```python
from build123d import *

# Parameters (mm, degrees)
SKETCH_R             = 2.5
PAD_DEPTH            = 4.7
SKETCH_MIRRORED_2_R  = 2.5
PAD_MIRRORED_2_DEPTH = 4.7


with BuildPart() as part:
    # Sketch → Pad (new body)
    with BuildSketch(Plane.XY):
        with BuildLine():
            Line((0, 0), (28.25, 0))
            Line((28.25, 0), (28.25, 23.538582))
            ThreePointArc((28.25, 23.538582), (26.870058, 26.870058), (23.538582, 28.25))
            Line((23.538582, 28.25), (0, 28.25))
            Line((0, 28.25), (0, 0))
        make_face()
        with Locations((23.5, 23.5)):
            Circle(SKETCH_R, mode=Mode.SUBTRACT)
    pad = extrude(amount=PAD_DEPTH)

    # Sketch Mirrored 2 → Pad Mirrored 2 (add)
    with BuildSketch(Plane(origin=(0, 0, 0), x_dir=(-1, 0, 0), z_dir=(0, 0, -1))):
        with BuildLine():
            Line((0, 0), (28.25, 0))
            Line((28.25, 0), (28.25, 23.538582))
            ThreePointArc((28.25, 23.538582), (26.870058, 26.870058), (23.538582, 28.25))
            Line((23.538582, 28.25), (0, 28.25))
            Line((0, 28.25), (0, 0))
        make_face()
        with Locations((23.5, 23.5)):
            Circle(SKETCH_MIRRORED_2_R, mode=Mode.SUBTRACT)
    pad_mirrored_2 = extrude(amount=-PAD_MIRRORED_2_DEPTH)

    # Mirrored001: Pad, Pad Mirrored 2 across Sketch H_Axis
    add(pad.mirror(Plane.ZX))
    add(pad_mirrored_2.mirror(Plane.ZX))

    # Sketch001 → Revolution (revolve)
    with BuildSketch(Plane.XZ):
        Polygon((19, 0), (28.25, 0), (28.25, 14.5), (27.5, 14.5), (27.5, 51), (28.25, 51), (28.25, 67), (0, 67), (0, -1.5), (19, -1.5), align=None)
    revolve(axis=Axis((0, 0, 0), (0, 0, 1)))


solid = part.part
```
Input: part model. Units: mm. Frame: model coordinates. A direction names the side the tool comes from. Give positions to 0.01 mm unless a question says otherwise; leave off trailing zeros. Loops run counter-clockwise (first coordinate to the right, second up) from the corner with the lowest first, then second, coordinate; pieces in that order, holes last.
1) Line query: L1, parallel to Y at x = -23.5, z = 2.05; L2, parallel to Y at x = -23, z = 2. Output: solid intervals per line, ascending.
A:
L1: y = -28.25 to -26, -21 to 21, 26 to 28.25
L2: y = -28.25 to -25.95, -21.05 to 21.05, 25.95 to 28.25
2) Reachability of faces 4 (the flat face through (-21, -22, 4.7)), 5 (the cylindrical face through (8.767, -16.856, -0.74)), 6 (the flat face through (0, 0, 67)), 7 (the flat face through (-6, -27, 51)), 8 (the cylindrical face through (15.19, 23.82, 9.67)) from +Z, -Z, +X, -X, +Y, -Y: full face, straight path, thin tool, end or side. Return the list, or none.
A:
face 4: +Z, -X, -Y
face 5: -Z
face 6: +Z, +X, -X, +Y, -Y
face 7: none
face 8: +Z
3) Section query A-A on x = 13. Return the cut outline in (y, z), and give its area (3 significant figures).
A:
outline: (-28.25, 0) - (-13.86, 0) - (-13.86, -1.5) - (13.86, -1.5) - (13.86, 0) - (28.25, 0) - (28.25, 4.7) - (25.08, 4.7) - (25.08, 14.5) - (24.23, 14.5) - (24.23, 51) - (25.08, 51) - (25.08, 67) - (-25.08, 67) - (-25.08, 51) - (-24.23, 51) - (-24.23, 14.5) - (-25.08, 14.5) - (-25.08, 4.7) - (-28.25, 4.7) - close
area: 3,370 mm2
4) Section query C-C on z = 29. Return the cut outline in (x, y), and give its area (3 significant figures).
A:
outline: circle Ø55 at (0, 0)
area: 2,380 mm2
5) Contact query for flat-ended pins moving along their axis: pin 1 (10 mm diameter, centred on x = 16.5, z = 20, fed in from -Y); pin 2 (2 mm diameter, centred on y = -19.5, z = 23.5, fed in from -X); pin 3 (1 mm diameter, centred on y = -4, z = 60, fed in from -X). Output: stop coordinate, or through.
A:
pin 1: stops at y = -24.98
pin 2: stops at x = -20.35
pin 3: stops at x = -28.03
6) Section query D-D on z = 63. Return the cut outline in (x, y).
A:
outline: circle Ø56.5 at (0, 0)
7) Mould query, pull axis Z, two halves, no side actions, for faces 1 (the cylindrical face through (-5.961, -26.846, 33.006)), 2 (the flat face through (21.5, -21.5, 4.7)), 3 (the cylindrical face through (21.66, -25.19, 2.32)). Classes: released by +Z, released by -Z, zero draft, split by the parting line, or undercut.
A:
face 1: undercut
face 2: released by +Z
face 3: zero draft
